Can you work these out from the model? Positions are in its coordinate system, mm. Face numbers are marked on the shaded views. Round coordinates to 2 decimals unless told otherwise and drop trailing zeros. Loops run counter-clockwise (first coordinate to the right, second up) from the corner with the lowest first, then second, coordinate; pieces in that order, holes last. Notation, with made-up numbers: (49, -28.5) -> (57, -28.5) arc R24 cw to (57, -17.5) -> close; hole circle Ø3 at (65.5, -20.75). An arc over 180 degrees is marked (long way). Write item = value, one per line.
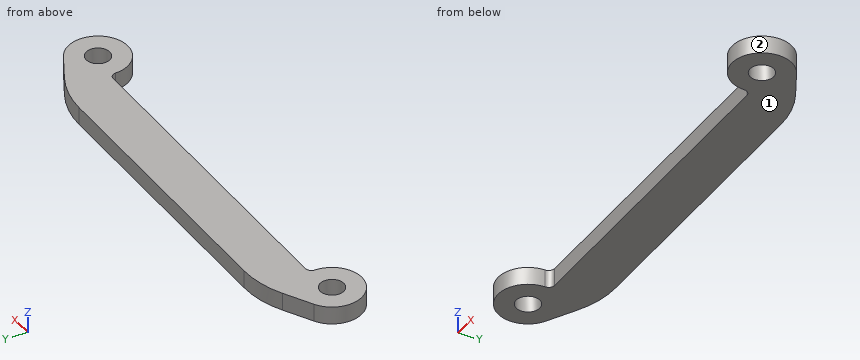
Autodesk Inventor part; units mm, degrees
ref_plane "YZ Plane" through (0, 0, 0) normal (1, 0, 0) x (0, 1, 0)
ref_plane "XZ Plane" through (0, 0, 0) normal (0, 1, 0) x (-1, 0, 0)
ref_plane "XY Plane" through (0, 0, 0) normal (0, 0, 1) x (1, 0, 0)
sketch "Sketch1" plane through (0, 0, 0) normal (0, 0, 1) x (1, 0, 0)
  line L0 (-22.225, 0) -> (22.225, 0)
  line L1 (-22.225, 0) -> (-28.8416, -3.6137)
  arc A0 (-28.8416, -3.6137) -> (-22.9235, -7.1247) centre (-26.924, -7.1247) ccw
  line L2 (-22.9235, -7.1247) -> (-22.9235, -6.35)
  circle A1 centre (-26.924, -7.1247) radius 1.5875
  line L3 (0, -15.1277) -> (0, 2.5213)
  line L4 (22.225, 0) -> (28.8416, -3.6137)
  arc A2 (22.9235, -7.1247) -> (28.8416, -3.6137) centre (26.924, -7.1247) ccw
  line L5 (22.9235, -7.1247) -> (22.9235, -6.35)
  circle A3 centre (26.924, -7.1247) radius 1.5875
  line L6 (-22.9235, -6.35) -> (22.9235, -6.35)
  point P0 (0, 0)
  point P1 (0, 0)
  point P2 (-26.924, -11.1252)
  point P3 (26.924, -11.1252)
  dimension "d0" = 8.001
  dimension "d1" = 3.175
  dimension "d2" = 4.7752
  dimension "d3" = 6.35
  dimension "d4" = 44.45
  dimension "d5" = 53.848
extrude "Extrusion1" add sketch "Sketch1" along normal mid plane 2.3813
fillet "Fillet1" radius 12.7 2 edges at (-22.225, 0, 0) (22.225, 0, 0)
fillet "Fillet2" radius 0.8128 2 edges at (-22.9235, -6.35, 0) (22.9235, -6.35, 0)
properties part number "Front Lower Arm Brace"
1. I'm going to push a flat-ended pin straight in: pin 1 (3 mm diameter, centred on x = -26.92, y = -7.12, fed in from +Z). Where does the tip first touch, or does it pass through?
Entries:
pin_1 = through
2. We'd pull the mould along X, two halves only. Please class the marked faces 1 and 2: released by +X, released by -X, zero draft, split by the parting line, or undercut.
Entries:
face_1 = zero draft
face_2 = undercut
3. Suppose I cut it at C-C, the plane x = 0.5. List the corners of the cut face in (y, z) for me.
Entries:
outline = (-6.35, -1.19) -> (0, -1.19) -> (0, 1.19) -> (-6.35, 1.19) -> close
4. Suppose I cut it at A-A, the plane y = -9.75. List the corners of the cut face in (x, z) for me, and give its area (3 significant figures).
Entries:
outline = (-29.94, -1.19) -> (-23.91, -1.19) -> (-23.91, 1.19) -> (-29.94, 1.19) -> close; (23.91, -1.19) -> (29.94, -1.19) -> (29.94, 1.19) -> (23.91, 1.19) -> close
area = 28.8 mm²
5. I need wall thicknesses on line 1 (X direction, y = -6, z = 0.3); line 2 (X direction, y = -7.75, z = -0.55); line 3 (Y direction, x = 0, z = -0.3). Which ranges of each line are inside material? Lowest first, please. Write a range as [from, to].
Entries:
line_1 = [-30.76, -28.04], [-25.8, 25.8], [28.04, 30.76]
line_2 = [-30.88, -28.38], [-25.46, -22.97], [22.97, 25.46], [28.38, 30.88]
line_3 = [-6.35, 0]
6. Suppose I cut it at B-B, the plane z = 0.1. Count the separate pieces of the cut face and the enclosed holes in it, and give its area (3 significant figures).
Entries:
separate_pieces = 1
enclosed_holes = 2
area = 395 mm²
7. Suppose I cut it at D-D, the plane y = -2.25. List the corners of the cut face in (x, z) for me, and give its area (3 significant figures).
Entries:
outline = (-26.34, -1.19) -> (26.34, -1.19) -> (26.34, 1.19) -> (-26.34, 1.19) -> close
area = 125 mm²
